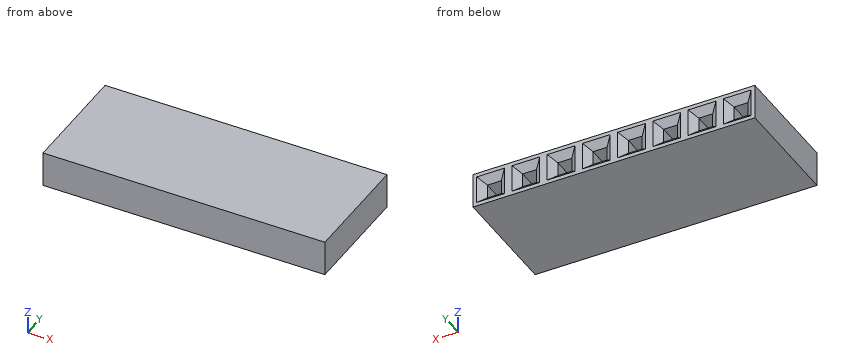
from build123d import *

# Parameters (mm, degrees)
SKETCH1_W                  = 2.54
SKETCH1_H                  = 2.54
BOSS_EXTRUDE1_DEPTH        = 8.3
SKETCH2_W                  = 1
SKETCH2_H                  = 1
CUT_EXTRUDE1_DEPTH         = 4
CHAMFER1_SIZE              = 0.5
LPATTERN1_COUNT            = 8
LPATTERN1_PITCH            = 2.54
CHAMFER1_OF_LPATTERN1_SIZE = 0.5


with BuildPart() as part:
    # Sketch1 → Boss-Extrude1 (new body)
    with BuildSketch(Plane(origin=(0, 0, 0), x_dir=(1, 0, 0), z_dir=(0, 1, 0))):
        Rectangle(SKETCH1_W, SKETCH1_H)
    boss_extrude1 = extrude(amount=BOSS_EXTRUDE1_DEPTH)

    # Sketch2 → Cut-Extrude1 (cut)
    with BuildSketch(Plane(origin=(0, 8.3, 0), x_dir=(-1, 0, 0), z_dir=(0, 1, 0))):
        Rectangle(SKETCH2_W, SKETCH2_H)
    cut_extrude1 = extrude(amount=-CUT_EXTRUDE1_DEPTH, mode=Mode.SUBTRACT)

    # Chamfer1
    chamfer1_edges = [part.edges().sort_by_distance(p)[0] for p in [
        (0, 8.3, 0.5),
        (0.5, 8.3, 0),
        (0, 8.3, -0.5),
        (-0.5, 8.3, 0),
    ]]
    chamfer(chamfer1_edges, length=CHAMFER1_SIZE)

    # LPattern1: Boss-Extrude1, Cut-Extrude1 ×8
    with Locations(*[(i * LPATTERN1_PITCH, 0, 0) for i in range(1, LPATTERN1_COUNT)]):
        add(boss_extrude1)
        add(cut_extrude1, mode=Mode.SUBTRACT)

    # Chamfer1 of LPattern1
    chamfer1_of_lpattern1_edges = [part.edges().sort_by_distance(p)[0] for p in [
        (2.54, 8.3, 0.5),
        (3.04, 8.3, 0),
        (2.54, 8.3, -0.5),
        (2.04, 8.3, 0),
        (5.08, 8.3, 0.5),
        (5.58, 8.3, 0),
        (5.08, 8.3, -0.5),
        (4.58, 8.3, 0),
        (7.62, 8.3, 0.5),
        (8.12, 8.3, 0),
        (7.62, 8.3, -0.5),
        (7.12, 8.3, 0),
        (10.16, 8.3, 0.5),
        (10.66, 8.3, 0),
        (10.16, 8.3, -0.5),
        (9.66, 8.3, 0),
        (12.7, 8.3, 0.5),
        (13.2, 8.3, 0),
        (12.7, 8.3, -0.5),
        (12.2, 8.3, 0),
        (15.24, 8.3, 0.5),
        (15.74, 8.3, 0),
        (15.24, 8.3, -0.5),
        (14.74, 8.3, 0),
        (17.78, 8.3, 0.5),
        (18.28, 8.3, 0),
        (17.78, 8.3, -0.5),
        (17.28, 8.3, 0),
    ]]
    chamfer(chamfer1_of_lpattern1_edges, length=CHAMFER1_OF_LPATTERN1_SIZE)


solid = part.part
CAD build for the part. Positions are in the model's coordinates, mm. Round coordinates to 2 decimals unless told otherwise and drop trailing zeros. Loops run counter-clockwise (first coordinate to the right, second up) from the corner with the lowest first, then second, coordinate; pieces in that order, holes last. Notation, with made-up numbers: (29.25, 56.25) - (73.25, 56.25) arc R16 ccw to (73.25, 65.25) - close; hole circle Ø9 at (30.5, -5.5). An arc over 180 degrees is marked (long way). Put each result on its own line as item: value.
1. Wall check: line 1 (Y direction, x = 7.5, z = -0.45); line 2 (Y direction, x = 13.5, z = -0.1). Give the ranges that are in metal, low to high.
Geometry check:
line 1: 0 to 4.3
line 2: 0 to 8.1
2. Slice it at B-B on y = 6.5. Give the number of separate pieces and of enclosed holes in the cut face, and give its area (3 significant figures).
Geometry check:
separate pieces: 1
enclosed holes: 8
area: 43.6 mm²
3. Pin check, flat tips, straight feed: P1, Ø0.8, axis at x = 0, z = 0, coming from the +Y side; P2, Ø1.1, axis at x = 12.5, z = 0, coming from the +Y side; P3, Ø1.1, axis at x = 2.5, z = 0, coming from the +Y side. Stop position of each tip, or through.
Geometry check:
P1: y = 4.3
P2: y = 8.05
P3: y = 7.89
4. Slice it at A-A on x = 10.25. List the corners of the cut face in (y, z).
Geometry check:
outline: (0, -1.27) - (8.3, -1.27) - (8.3, -1) - (7.8, -0.5) - (4.3, -0.5) - (4.3, 0.5) - (7.8, 0.5) - (8.3, 1) - (8.3, 1.27) - (0, 1.27) - close
